Source: CAD feature listing. Evaluate the final solid. Frame: model axes, mm. A direction names the side the tool comes from. Give positions to 0.01 mm unless a question says otherwise; leave off trailing zeros. Order: outer loops, then holes, each group sorted by start corner. A loop starts at its lowest first (then second) coordinate and runs counter-clockwise, first axis right, second up.
from build123d import *

# Parameters (mm, degrees)
SKETCH1_W             = 114
SKETCH1_H             = 50
BOSS_EXTRUDE1_DEPTH   = 4.75
SKETCH2_R             = 8
CUT_EXTRUDE1_DEPTH    = 63.962290301
FILLET1_R             = 5
SKETCH3_R             = 5
CUT_EXTRUDE2_DEPTH    = 4
SKETCH4_R             = 3
CUT_EXTRUDE3_DEPTH    = 63.483997951
M4_TAPPED_HOLE1_D     = 3.3
M4_TAPPED_HOLE2_D     = 3.3
M4_TAPPED_HOLE2_DEPTH = 14.1
M4_TAPPED_HOLE2_TIP   = 0.991420021


with BuildPart() as part:
    # Sketch1 → Boss-Extrude1 (new, symmetric)
    with BuildSketch(Plane.XY):
        Rectangle(SKETCH1_W, SKETCH1_H)
    extrude(amount=BOSS_EXTRUDE1_DEPTH, both=True)

    # Sketch2 → Cut-Extrude1 (cut, through all)
    with BuildSketch(Plane.XY.offset(4.75)):
        with BuildLine():
            Line((-37, -5), (-37, -25))
            Line((-37, -25), (13, -25))
            Line((13, -25), (13, -5))
            ThreePointArc((13, -5), (11.535533906, -1.464466094), (8, 0))
            Line((8, 0), (-32, 0))
            ThreePointArc((-32, 0), (-35.535533906, -1.464466094), (-37, -5))
        make_face()
        with BuildLine():
            Line((-57, -25), (-47, -25))
            Line((-47, -25), (-47, -5))
            ThreePointArc((-47, -5), (-48.464466094, -1.464466094), (-52, 0))
            Line((-52, 0), (-57, 0))
            Line((-57, 0), (-57, -25))
        make_face()
        with Locations((35, 12.5)):
            Circle(SKETCH2_R)
    extrude(amount=-CUT_EXTRUDE1_DEPTH, mode=Mode.SUBTRACT)

    # Fillet1
    fillet1_edges = [part.edges().sort_by_distance(p)[0] for p in [
        (57, 25, 0),
    ]]
    fillet(fillet1_edges, radius=FILLET1_R)

    # Sketch3 → Cut-Extrude2 (cut)
    with BuildSketch(Plane.XY.offset(4.75)):
        with Locations((-28.5, 12.5)):
            Circle(SKETCH3_R)
    extrude(amount=-CUT_EXTRUDE2_DEPTH, mode=Mode.SUBTRACT)

    # Sketch4 → Cut-Extrude3 (cut, through all)
    with BuildSketch(Plane.XY.offset(0.75)):
        with Locations((-28.5, 12.5)):
            Circle(SKETCH4_R)
    extrude(amount=-CUT_EXTRUDE3_DEPTH, mode=Mode.SUBTRACT)

    # M4 Tapped Hole1 (through all)
    with Locations(Plane.XY.offset(4.75)):
        with Locations((-46.77, 9.5), (-46.77, 16.5)):
            Hole(M4_TAPPED_HOLE1_D / 2)

    # M4 Tapped Hole2
    with Locations(Plane(origin=(0, -25, 0), x_dir=(-1, 0, 0), z_dir=(0, -1, 0))):
        with Locations((42, 0), (-21, 0), (-49, 0)):
            Hole(M4_TAPPED_HOLE2_D / 2, depth=M4_TAPPED_HOLE2_DEPTH)
            with Locations((0, 0, -(M4_TAPPED_HOLE2_DEPTH + M4_TAPPED_HOLE2_TIP / 2))):  # 118° drill point
                Cone(0, M4_TAPPED_HOLE2_D / 2, M4_TAPPED_HOLE2_TIP, mode=Mode.SUBTRACT)


solid = part.part
1) Section query B-B on y = 12.5. Output: boundary loops of the cut face in (x, z), and give its area (3 significant figures).
Checks:
outline: (-57, -4.75) - (-31.5, -4.75) - (-31.5, 0.75) - (-33.5, 0.75) - (-33.5, 4.75) - (-57, 4.75) - close; (-25.5, -4.75) - (27, -4.75) - (27, 4.75) - (-23.5, 4.75) - (-23.5, 0.75) - (-25.5, 0.75) - close; (43, -4.75) - (57, -4.75) - (57, 4.75) - (43, 4.75) - close
area: 858 mm2
2) Section query A-A on y = -15. Output: boundary loops of the cut face in (x, z).
Checks:
outline: (-47, -4.75) - (-37, -4.75) - (-37, 4.75) - (-47, 4.75) - close; (13, -4.75) - (57, -4.75) - (57, 4.75) - (13, 4.75) - close; hole circle Ø3.3 at (-42, 0); hole circle Ø3.3 at (21, 0); hole circle Ø3.3 at (49, 0)
3) Reachability of faces 1 (the face through (47.35, -17.85, -0.07)), 2 (the face through (-32.185, 15.879, 2.778)), 3 (the face through (-12, 0, 0)) from +Z, -Z, +X, -X, +Y, -Y: full face, straight path, thin tool, end or side. Return the list, or none.
Checks:
face 1: -Y
face 2: +Z
face 3: +Z, -Z, -Y
4) Ray query, L1, parallel to Z at x = 49, y = -17; L2, parallel to Y at x = -28.5, z = -2.95; L3, parallel to Y at x = -46.77, z = 2. Return the intervals inside material, ascending.
Checks:
L1: z = -4.75 to -1.65, 1.65 to 4.75
L2: y = 0 to 9.5, 15.5 to 25
L3: y = -25 to 7.85, 11.15 to 14.85, 18.15 to 25
5) First-contact query: pin 1 Ø1 at (y, z) = (-8, -3.5) entering from -X; pin 2 Ø3 at (x, z) = (-13, -1.5) entering from -Y; pin 3 Ø7 at (x, y) = (-28.5, 12.5) entering from +Z. Flat tips, straight axial feed; report the tip coordinate or a pass-through.
Checks:
pin 1: stops at x = -47
pin 2: stops at y = 0
pin 3: stops at z = 0.75
6) Section query C-C on y = 6. Output: boundary loops of the cut face in (x, z).
Checks:
outline: (-57, -4.75) - (30.34, -4.75) - (30.34, 4.75) - (-57, 4.75) - close; (39.66, -4.75) - (57, -4.75) - (57, 4.75) - (39.66, 4.75) - close
7) Pull-direction query (X, two-part tool) for faces 4 (the face through (-37, -15, 0)), 5 (the face through (-47, -15, 0)), 6 (the face through (-1, 6, -4.75)); classes: +X half, -X half, draft (parallel to the pull), parting line (faces both ways), or undercut.
Checks:
face 4: undercut
face 5: -X half
face 6: draft
